Autodesk Inventor part; units mm, degrees
ref_plane "YZ Plane" through (0, 0, 0) normal (1, 0, 0) x (0, 1, 0)
ref_plane "XZ Plane" through (0, 0, 0) normal (0, 1, 0) x (-1, 0, 0)
ref_plane "XY Plane" through (0, 0, 0) normal (0, 0, 1) x (1, 0, 0)
sketch "Sketch1" plane through (0, 0, 0) normal (0, 0, 1) x (1, 0, 0)
  line L0 (0, 0) -> (214.63, 0)
  line L1 (214.63, 0) -> (214.63, 146.05)
  line L2 (214.63, 146.05) -> (0, 146.05)
  line L3 (0, 146.05) -> (0, 0)
  line L4 (0, 146.05) -> (-6.35, 146.05) construction
  line L5 (-6.35, 146.05) -> (-6.35, 0) construction
  line L6 (-6.35, 0) -> (0, 0) construction
  line L7 (214.63, 0) -> (220.98, 0) construction
  line L8 (220.98, 0) -> (220.98, 146.05) construction
  line L9 (214.63, 146.05) -> (220.98, 146.05) construction
  line L10 (-8.255, 0) -> (-8.255, 93.2539)
  line L11 (222.885, 0) -> (222.885, 86.8023)
  line L12 (-8.255, 0) -> (222.885, 0)
  point P0 (-3.175, 146.05)
  point P1 (217.805, 146.05)
  point P2 (107.315, 0)
  dimension "d0" = 146.05
  dimension "d1" = 214.63
  dimension "d17" = 6.35
  dimension "d18" = 6.35
  dimension "d19" = 227.33
  dimension "d21" = 220.98
  dimension "d56" = 5.08
  dimension "d57" = 231.14
extrude "Extrusion1" add sketch "Sketch1" along normal mid plane 6.35
sketch "Sketch2" plane through (0, 0, 3.175) normal (0, 0, 1) x (1, 0, 0)
  circle A0 centre (11.5378, 135.236) radius 2
  circle A1 centre (11.5378, 36.736) radius 2
  line L0 (6.6378, 141.986) -> (16.4378, 141.986) construction
  line L1 (16.4378, 141.986) -> (16.4378, 29.986) construction
  line L2 (16.4378, 29.986) -> (6.6378, 29.986) construction
  line L3 (6.6378, 29.986) -> (6.6378, 141.986) construction
  line L4 (11.5378, 36.736) -> (11.5378, 135.236) construction
  line L5 (0, 0) -> (214.63, 0) construction
  line L6 (0, 146.05) -> (0, 0)
  line L7 (-6.35, 146.05) -> (-6.35, 0) construction
  line L8 (6.6378, 128.336) -> (8.2378, 128.336) construction
  line L9 (8.2378, 128.336) -> (8.2378, 43.636) construction
  line L10 (8.2378, 43.636) -> (6.6378, 43.636) construction
  line L11 (6.6378, 43.636) -> (6.6378, 128.336) construction
  line L12 (16.4378, 128.336) -> (14.8378, 128.336) construction
  line L13 (14.8378, 128.336) -> (14.8378, 43.636) construction
  line L14 (14.8378, 43.636) -> (16.4378, 43.636) construction
  line L15 (16.4378, 43.636) -> (16.4378, 128.336) construction
  line L16 (214.63, 146.05) -> (0, 146.05)
  line L17 (-8.255, 0) -> (-8.255, 93.2539)
  point P0 (11.5378, 141.986)
  point P1 (11.5378, 85.986)
  point P2 (16.4378, 85.986)
  point P3 (14.8378, 85.986)
  point P4 (8.2378, 85.986)
  dimension "d4" = 98.5
  dimension "d5" = 4
  dimension "d7" = 9.8
  dimension "d8" = 141.986
  dimension "d22" = 112
  dimension "d23" = 6.6
  dimension "d24" = 13.65
  dimension "d58" = 19.7928
extrude "Extrusion2" cut sketch "Sketch2" against normal blind 9.525
pattern_linear "Rectangular Pattern1" count 12 spacing 17.78 along (1, 0, 0) of "Extrusion2"
sketch "Sketch3" plane through (0, 0, 3.175) normal (0, 0, 1) x (1, 0, 0)
  line L0 (12.7, 44.45) -> (201.93, 44.45)
  line L1 (201.93, 44.45) -> (201.93, 127)
  line L2 (201.93, 127) -> (12.7, 127)
  line L3 (12.7, 127) -> (12.7, 44.45)
  line L4 (214.63, 0) -> (214.63, 146.05)
  line L5 (0, 146.05) -> (0, 0)
  line L6 (214.63, 146.05) -> (0, 146.05)
  line L7 (0, 0) -> (214.63, 0)
  dimension "d49" = 12.7
  dimension "d50" = 12.7
  dimension "d51" = 19.05
  dimension "d52" = 44.45
extrude "Extrusion3" cut sketch "Sketch3" against normal through all contours L3 L2 L1 L0
fillet "Fillet1" radius 3.175 4 edges at (12.7, 44.45, 0) (12.7, 127, 0) (201.93, 44.45, 0) (201.93, 127, 0)
sketch "Sketch5" plane through (0, 0, 3.175) normal (0, -1, 0) x (1, 0, 0)
  line L0 (0, -6.35) -> (0, 0)
  point P0 (0, -3.175)
  point P1 (67.945, -3.175)
  point P2 (0, -3.175)
  point P3 (-8.255, -3.175)
  point P4 (-8.255, -3.175)
  point P5 (-8.255, -3.175)
  point P6 (139.065, -3.175)
  point P7 (0, -3.175)
  dimension "d69" = 76.2
  dimension "d70" = 147.32
hole "Hole1" at (67.945, 0, 0) at (139.065, 0, 0) direction (0, 1, 0) diameter 3.9688 depth 9.525 tip angle 118
equation "\"d18\" = d17"
properties part number "Center Wall" material "ABS Plastic"
Geometry check sheet. Reference: the model listing, model coordinates, mm. Give positions to 0.01 mm unless a question says otherwise; leave off trailing zeros. Write each loop counter-clockwise with the first axis right and the second up, starting at its lowest first coordinate (ties: lowest second). Pieces come first, ordered by that corner, then holes.
1) Release check for a two-part mould opening along Z. For faces 1 (the cylindrical face through (116.22, 135.32, 0.04)), 2 (the cylindrical face through (140.826, 4.829, -0.916)) record: pulls with the +Z half, pulls with the -Z half, needs draft (parallel to the pull), parting line crosses it, or undercut.
2) Section check A-A, the plane x = 37.5. Record the boundary of the cut face in (y, z) (3 decimals), and give its area (3 significant figures).
3) Section check B-B, the plane y = 59.5. Record the boundary of the cut face in (x, z) (3 decimals).
4) Material ranges on L1, parallel to X at y = 66.5, z = 0.75; L2, parallel to Y at x = 52.5, z = 2.25; L3, parallel to Y at x = 101, z = 1.25, recorded low to high.
Computed:
1. face 1: needs draft
1. face 2: undercut
2. outline: (0, -3.175) - (44.45, -3.175) - (44.45, 3.175) - (0, 3.175) - close; (127, -3.175) - (146.05, -3.175) - (146.05, 3.175) - (127, 3.175) - close
2. area: 403 mm2
3. outline: (0, -3.175) - (12.7, -3.175) - (12.7, 3.175) - (0, 3.175) - close; (201.93, -3.175) - (214.63, -3.175) - (214.63, 3.175) - (201.93, 3.175) - close
4. L1: x = 0 to 12.7, 201.93 to 214.63
4. L2: y = 0 to 44.45, 127 to 146.05
4. L3: y = 0 to 34.82, 38.66 to 44.45, 127 to 133.32, 137.16 to 146.05
